from build123d import *

# Parameters (mm, degrees)
EXTRUDE_1_DEPTH     = 60
EXTRUDE_2_DEPTH     = 9
SKETCH_7_R          = 11
EXTRUDE_3_DEPTH     = 2
SKETCH_8_R          = 2.5
EXTRUDE_4_DEPTH     = 18
CUT_EXTRUDE_START   = -15
CUT_EXTRUDE_1_DEPTH = 15
SKETCH_10_R         = 1.6
CUT_EXTRUDE_2_DEPTH = 4.5
EXTRUDE_5_DEPTH     = 5
CUT_EXTRUDE_3_DEPTH = 5
SKETCH_13_R         = 0.562342784
EXTRUDE_6_DEPTH     = 5
SKETCH_14_R         = 2
SKETCH_14_R_2       = 1.75
CUT_EXTRUDE_4_DEPTH = 1


with BuildPart() as part:
    # 草图2 → 凸台-拉伸1 (new body)
    with BuildSketch(Plane(origin=(0, 0, 0), x_dir=(1, 0, 0), z_dir=(0, 1, 0))):
        Polygon((-14.012734328, 22.447763171), (-21.08380214, 15.376695359), (-21.08380214, -12.681169017), (-14.012734328, -19.752236829), (14.045130048, -19.752236829), (21.11619786, -12.681169017), (21.11619786, 15.376695359), (14.045130048, 22.447763171), align=None)
    extrude(amount=EXTRUDE_1_DEPTH)

    # 草图5 → 凸台-拉伸2 (add)
    with BuildSketch(Plane(origin=(0, 60, 0), x_dir=(1, 0, 0), z_dir=(0, 1, 0))):
        with BuildLine():
            Line((-16.776242784, 22.447763171), (16.776242784, 22.447763171))
            ThreePointArc((16.776242784, 22.447763171), (19.070321818, 20.399669839), (21.11619786, 18.103613191))
            Line((21.11619786, 18.103613191), (21.11619786, -15.408086849))
            ThreePointArc((21.11619786, -15.408086849), (19.070321818, -17.704143498), (16.776242784, -19.752236829))
            Line((16.776242784, -19.752236829), (-16.776242784, -19.752236829))
            ThreePointArc((-16.776242784, -19.752236829), (-19.051917848, -17.722547478), (-21.08380214, -15.448831998))
            Line((-21.08380214, -15.448831998), (-21.08380214, 18.14435834))
            ThreePointArc((-21.08380214, 18.14435834), (-19.051917848, 20.41807382), (-16.776242784, 22.447763171))
        make_face()
    extrude_2 = extrude(amount=-EXTRUDE_2_DEPTH)

    # 镜向1: 凸台-拉伸2 across plane
    add(extrude_2.mirror(Plane.ZX.offset(30)))

    # 草图7 → 凸台-拉伸3 (add)
    with BuildSketch(Plane(origin=(0, 60, 0), x_dir=(1, 0, 0), z_dir=(0, 1, 0))):
        with Locations(Location((0, 1.347763171, 0), (0, 0, 270))):
            Circle(SKETCH_7_R)
    extrude(amount=EXTRUDE_3_DEPTH)

    # 草图8 → 凸台-拉伸4 (add)
    with BuildSketch(Plane(origin=(0, 62, 0), x_dir=(1, 0, 0), z_dir=(0, 1, 0))):
        with Locations(Location((0, 1.347763171, 0), (0, 0, 270))):
            Circle(SKETCH_8_R)
    extrude(amount=EXTRUDE_4_DEPTH)

    # 草图9 → 切除-拉伸1 (cut)
    with BuildSketch(Plane(origin=(0, 80, 0), x_dir=(1, 0, 0), z_dir=(0, 1, 0)).offset(CUT_EXTRUDE_START)):
        with BuildLine():
            Line((-1.785357107, 3.097763171), (1.785357107, 3.097763171))
            ThreePointArc((1.785357107, 3.097763171), (0, 3.847763171), (-1.785357107, 3.097763171))
        make_face()
    extrude(amount=CUT_EXTRUDE_1_DEPTH, mode=Mode.SUBTRACT)

    # 草图10 → 切除-拉伸2 (cut)
    with BuildSketch(Plane(origin=(0, 60, 0), x_dir=(1, 0, 0), z_dir=(0, 1, 0))):
        with Locations(Location((-15.5, 16.847763171, 0), (0, 0, 270))):
            Circle(SKETCH_10_R)
        with Locations(Location((15.5, 16.847763171, 0), (0, 0, 270))):
            Circle(SKETCH_10_R)
        with Locations(Location((15.5, -14.152236829, 0), (0, 0, 270))):
            Circle(SKETCH_10_R)
        with Locations(Location((-15.5, -14.152236829, 0), (0, 0, 270))):
            Circle(SKETCH_10_R)
    extrude(amount=-CUT_EXTRUDE_2_DEPTH, mode=Mode.SUBTRACT)

    # 草图11 → 凸台-拉伸5 (add)
    with BuildSketch(Plane(origin=(0, 0, -22.447763171), x_dir=(-1, 0, 0), z_dir=(0, 0, -1))):
        Polygon((10, 0), (-10, 0), (-10, 5), (-9, 5), (-9, 1), (9, 1), (9, 5), (10, 5), align=None)
    extrude(amount=EXTRUDE_5_DEPTH)

    # 草图12 → 切除-拉伸3 (cut)
    with BuildSketch(Plane.XZ):
        Polygon((-7.144738058, -27.447763171), (-7.144738058, -24.447763171), (-7.644738058, -24.447763171), (-7.644738058, -26.447763171), (-8.144738058, -26.447763171), (-7.644738058, -27.447763171), align=None)
        Polygon((7.644738058, -27.447763171), (7.144738058, -27.447763171), (7.144738058, -24.447763171), (7.644738058, -24.447763171), (7.644738058, -26.447763171), (8.144738058, -26.447763171), align=None)
    extrude(amount=-CUT_EXTRUDE_3_DEPTH, mode=Mode.SUBTRACT)

    # 草图13 → 凸台-拉伸6 (add)
    with BuildSketch(Plane(origin=(0, 0, -22.447763171), x_dir=(-1, 0, 0), z_dir=(0, 0, -1))):
        with Locations(Location((-1.27, 3.54, 0), (0, 0, 180))):
            Circle(SKETCH_13_R)
        with Locations(Location((-3.81, 3.54, 0), (0, 0, 180))):
            Circle(SKETCH_13_R)
        with Locations(Location((-6.35, 3.54, 0), (0, 0, 180))):
            Circle(SKETCH_13_R)
        with Locations(Location((6.35, 3.54, 0), (0, 0, 180))):
            Circle(SKETCH_13_R)
        with Locations(Location((3.81, 3.54, 0), (0, 0, 180))):
            Circle(SKETCH_13_R)
        with Locations(Location((1.27, 3.54, 0), (0, 0, 180))):
            Circle(SKETCH_13_R)
    extrude(amount=EXTRUDE_6_DEPTH)

    # 草图14 → 切除-拉伸4 (cut)
    # profile 1 of 4: a face of its own
    with BuildSketch(Plane.XZ):
        with Locations(Location((14.11619786, 12.752236829, 0), (0, 0, 270))):
            Circle(SKETCH_14_R)
        with Locations(Location((14.11619786, 12.752236829, 0), (0, 0, 270))):
            Circle(SKETCH_14_R_2, mode=Mode.SUBTRACT)
    # profile 2 of 4: a face of its own
    with BuildSketch(Plane.XZ):
        with Locations(Location((12.752236829, -14.11619786, 0), (0, 0, 270))):
            Circle(SKETCH_14_R)
        with Locations(Location((12.752236829, -14.11619786, 0), (0, 0, 270))):
            Circle(SKETCH_14_R_2, mode=Mode.SUBTRACT)
    # profile 3 of 4: a face of its own
    with BuildSketch(Plane.XZ):
        with Locations(Location((-14.11619786, -12.752236829, 0), (0, 0, 270))):
            Circle(SKETCH_14_R)
        with Locations(Location((-14.11619786, -12.752236829, 0), (0, 0, 270))):
            Circle(SKETCH_14_R_2, mode=Mode.SUBTRACT)
    # profile 4 of 4: a face of its own
    with BuildSketch(Plane.XZ):
        with Locations(Location((-12.752236829, 14.11619786, 0), (0, 0, 270))):
            Circle(SKETCH_14_R)
        with Locations(Location((-12.752236829, 14.11619786, 0), (0, 0, 270))):
            Circle(SKETCH_14_R_2, mode=Mode.SUBTRACT)
    extrude(amount=-CUT_EXTRUDE_4_DEPTH, mode=Mode.SUBTRACT)


solid = part.part
Can you work these out from the model? Positions are in its coordinate system, mm. A direction names the side the tool comes from. Give positions to 0.01 mm unless a question says otherwise; leave off trailing zeros. Loops run counter-clockwise (first coordinate to the right, second up) from the corner with the lowest first, then second, coordinate; pieces in that order, holes last. Notation, with made-up numbers: M -16,80.5 L 14,80.5 A24 ccw 14,106.5 Z; hole C 38.25,83.25 d1. An arc over 180 degrees is marked long. One line per item, written item: value.
1) On a 3-axis mill with a long thin cutter (end or side, diameter ignored), from which of +Z, -Z, +X, -X, +Y, -Y can I reach the whole of each face in a straight line? I mean faces 1 (the face through (18, 9, 17)), 2 (the face through (9, 3, -25)), 3 (the face through (16.58, 57.78, -18.03)). Say none if no direction works.
Geometry check:
face 1: +Z, +X
face 2: -Z, +Y
face 3: +Y
2) Imagine slicing it at C-C on y = 67.5. Write out the boundary of the cut face in (x, z), and give its area (3 significant figures).
Geometry check:
outline: M -1.79,-3.1 L 1.79,-3.1 A2.5 ccw long Z
area: 17.8 mm²
3) Thinking about a two-plate mould opening in Z: for faces 4 (the face through (12.4, 0.5, 13.1)), 5 (the face through (16, 55.5, 14)), 6 (the face through (-19.022, 4.437, 17.753)), 7 (the face through (-17.5, 29.71, -18.96)), which applies, +Z half, -Z half, draft (parallel to the pull), parting line (faces both ways), or undercut?
Geometry check:
face 4: undercut
face 5: undercut
face 6: +Z half
face 7: -Z half
4) I'm going to push flat-ended pins straight in: pin 1 (0.8 mm diameter, centred on y = 0.5, z = -26, fed in from -X); pin 2 (2.5 mm diameter, centred on x = -1, z = -25, fed in from +Y); pin 3 (1.1 mm diameter, centred on x = 9.5, z = -24.5, fed in from +Y). Where does each tip first touch, or does it pass through?
Geometry check:
pin 1: stops at x = -10
pin 2: stops at y = 4.1
pin 3: stops at y = 5
5) Imagine slicing it at A-A on y = 31. Write out the boundary of the cut face in (x, z).
Geometry check:
outline: M -21.08,-15.38 L -14.01,-22.45 L 14.05,-22.45 L 21.12,-15.38 L 21.12,12.68 L 14.05,19.75 L -14.01,19.75 L -21.08,12.68 Z
6) Please list where these lines run through material, in increasing order: line 1 (Z direction, x = -15, y = 57); line 2 (Z direction, x = -14, y = 30); line 3 (Y direction, x = 17, z = -21.5).
Geometry check:
line 1: z = -22.45 to -18.37, -15.33 to 12.63, 15.67 to 19.75
line 2: z = -22.45 to 19.75
line 3: y = 0 to 9, 51 to 60
7) Imagine slicing it at B-B on z = 8. Write out the boundary of the cut face in (x, y), and give its area (3 significant figures).
Geometry check:
outline: M -21.08,0 L 21.12,0 L 21.12,60 L 5.8,60 L 5.8,62 L -5.8,62 L -5.8,60 L -21.08,60 Z
area: 2,560 mm²
